```python
from build123d import *

# Parameters (mm, degrees)
SKETCH_1_R      = 0.9
EXTRUDE_1_DEPTH = 2


with BuildPart() as part:
    # 草图1 → 凸台-拉伸1 (new body)
    with BuildSketch(Plane.XY):
        with BuildLine():
            Line((8.485281374, -5), (10.657359313, -5))
            ThreePointArc((10.657359313, -5), (11.80540961, -5.228361402), (12.778679656, -5.878679656))
            Line((12.778679656, -5.878679656), (13.9, -7))
            Line((13.9, -7), (18.9, -7))
            Line((18.9, -7), (18.9, -5.25))
            ThreePointArc((18.9, -5.25), (18.723223305, -4.823223305), (19.15, -5))
            Line((19.15, -5), (20.75, -5))
            ThreePointArc((20.75, -5), (21.176776695, -4.823223305), (21, -5.25))
            Line((21, -5.25), (21, -7))
            Line((21, -7), (23, -7))
            Line((23, -7), (23, 7))
            Line((23, 7), (21, 7))
            Line((21, 7), (21, 5.25))
            ThreePointArc((21, 5.25), (21.176776695, 4.823223305), (20.75, 5))
            Line((20.75, 5), (19.15, 5))
            ThreePointArc((19.15, 5), (18.723223305, 4.823223305), (18.9, 5.25))
            Line((18.9, 5.25), (18.9, 7))
            Line((18.9, 7), (13.9, 7))
            Line((13.9, 7), (12.778679656, 5.878679656))
            ThreePointArc((12.778679656, 5.878679656), (11.80540961, 5.228361402), (10.657359313, 5))
            Line((10.657359313, 5), (8.485281374, 5))
            ThreePointArc((8.485281374, 5), (7.632478509, 5.190931933), (6.942502943, 5.727272727))
            ThreePointArc((6.942502943, 5.727272727), (3.837612894, 8.140806304), (0, 9))
            ThreePointArc((0, 9), (-2.25, 6.75), (0, 4.5))
            ThreePointArc((0, 4.5), (4.5, 0), (0, -4.5))
            ThreePointArc((0, -4.5), (-2.25, -6.75), (0, -9))
            ThreePointArc((0, -9), (3.837612894, -8.140806304), (6.942502943, -5.727272727))
            ThreePointArc((6.942502943, -5.727272727), (7.632478509, -5.190931933), (8.485281374, -5))
        make_face()
        with Locations((0, 6.75)):
            Circle(SKETCH_1_R, mode=Mode.SUBTRACT)
        with Locations((0, -6.75)):
            Circle(SKETCH_1_R, mode=Mode.SUBTRACT)
        with Locations((11, 0)):
            Circle(SKETCH_1_R, mode=Mode.SUBTRACT)
    extrude(amount=EXTRUDE_1_DEPTH)


solid = part.part
```
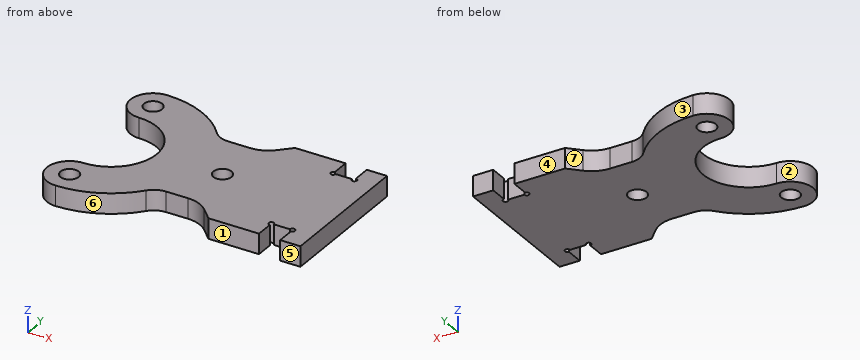
Part model, mm, in its own coordinate system. Face numbers are marked on the shaded views. A direction names the side the tool comes from. Round coordinates to 2 decimals unless told otherwise and drop trailing zeros. Loops run counter-clockwise (first coordinate to the right, second up) from the corner with the lowest first, then second, coordinate; pieces in that order, holes last. Notation, with made-up numbers: (39.25, 9.5) -> (86.25, 9.5) arc R17 cw to (86.25, 18.5) -> close; hole circle Ø1 at (-16.75, 36). An arc over 180 degrees is marked (long way). Use CSV: the item, a comma, the result in double quotes. Start each with the question number.
1) Pull direction X, two halves, no side cores. Call the marked faces 1, 2 and 3: +X half, -X half, draft (parallel to the pull), parting line (faces both ways), or undercut.
2) Which spindle directions (+Z, -Z, +X, -X, +Y, -Y) get a long thin tool onto all of the face, cutting with end or side? Do the marked faces 4, 5, 6 and 7. Say none if no direction does.
3) Cut at D-D, the plane y = 6.75. Write the cut outline in (x, z).
4) Cut at B-B, the plane z = 1.2. Give the number of separate pieces and of enclosed holes in the cut face, plus the area to 3 significant figures.
5) Cut at A-A, the plane y = 0. Write the cut outline in (x, z), plus the area to 3 significant figures.
6) Drop flat-ended pins along their axis: P1, Ø0.9, axis at y = 6, z = 1, coming from the -X side; P2, Ø1, axis at x = 15.5, z = 1, coming from the +Y side; P3, Ø1.4, axis at x = 11, y = 0, coming from the -Z side; P4, Ø1, axis at x = 10, z = 1.5, coming from the +Y side. Give the stop position or say it passes through.
7) Wall check: L1, parallel to X at y = -6.25, z = 1.1; L2, parallel to Y at x = 8.75, z = 1.65; L3, parallel to X at y = 6.5, z = 1.8. Give the ranges that are in metal, low to high. Write a range as [from, to].
8) Cut at C-C, the plane x = 2. Write the cut outline in (y, z).
Determined:
1,face 1,"draft"
1,face 2,"-X half"
1,face 3,"undercut"
2,face 4,"+Z, -Z, +X, +Y"
2,face 5,"+Z, -Z, +X, -Y"
2,face 6,"+Z, -Z, -Y"
2,face 7,"+Z, -Z, +Y"
3,outline,"(-2.25, 0) -> (-0.9, 0) -> (-0.9, 2) -> (-2.25, 2) -> close; (0.9, 0) -> (5.95, 0) -> (5.95, 2) -> (0.9, 2) -> close; (13.65, 0) -> (18.9, 0) -> (18.9, 2) -> (13.65, 2) -> close; (21, 0) -> (23, 0) -> (23, 2) -> (21, 2) -> close"
4,separate pieces,"1"
4,enclosed holes,"3"
4,area,"281 mm2"
5,outline,"(4.5, 0) -> (10.1, 0) -> (10.1, 2) -> (4.5, 2) -> close; (11.9, 0) -> (23, 0) -> (23, 2) -> (11.9, 2) -> close"
5,area,"33.4 mm2"
6,P1,"stops at x = -2.23"
6,P2,"stops at y = 7"
6,P3,"passes through"
6,P4,"stops at y = 5"
7,L1,"x = [-2.19, -0.75], [0.75, 6.48], [13.15, 18.9], [21, 23]"
7,L2,"y = [-5, 5]"
7,L3,"x = [-2.24, -0.86], [0.86, 6.22], [13.4, 18.9], [21, 23]"
8,outline,"(-8.77, 0) -> (-4.03, 0) -> (-4.03, 2) -> (-8.77, 2) -> close; (4.03, 0) -> (8.77, 0) -> (8.77, 2) -> (4.03, 2) -> close"
